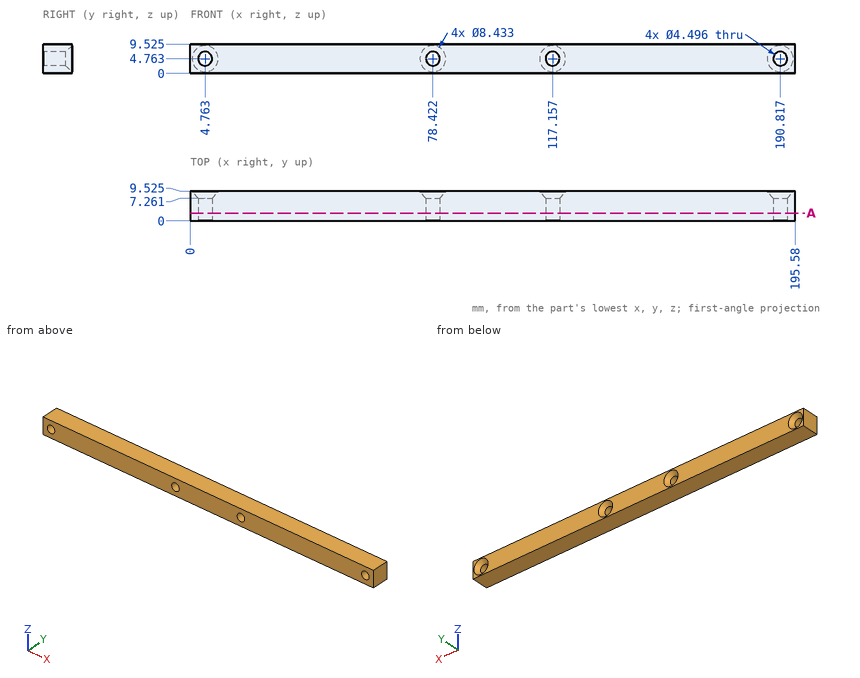
Verification items for this drawing (mm, ordinates from the low corner). Coordinates: 2 decimals unless noted, no trailing zeros. Order: outer loops, then holes, each group sorted by start corner. A loop starts at its lowest first (then second) coordinate and runs counter-clockwise, first axis right, second up. Notation, with made-up numbers: M 52.5,7.5 L 82.5,7.5 A29 ccw 82.5,40.5 Z; hole C 49.25,-25.5 d2. An arc over 180 degrees is marked long. Write each question's results on one line, items separated by ' | '.
1) Gauge pin test, flat ends, axial feed: pin 1 Ø5 at (x, z) = (22.5, 3.5) entering from -Y; pin 2 Ø5 at (x, z) = (78.42, 4.76) entering from +Y (1 decimal). Record the tip position at first contact, or that the pin passes through.
Solved:
pin 1: stops at y = 0 | pin 2: stops at y = 7.6
2) Scan lines: line 1 along X through (y, z) = (1.75, 3.5); line 2 along X through (y, z) = (5.5, 5.5) (1 decimal). Record each from-to range of solid material in increasing order. Write a range as [from, to].
Solved:
line 1: x = [0, 2.9], [6.62, 76.56], [80.28, 115.3], [119.02, 188.96], [192.68, 195.58] | line 2: x = [0, 2.6], [6.9, 76.3], [80.5, 115], [119.3, 188.7], [192.9, 195.6]
3) Section check A-A on y = 2.5. Record the cut outline in (x, z) (1 decimal).
Solved:
outline: M 0,0 L 195.6,0 L 195.6,9.5 L 0,9.5 Z; hole C 4.8,4.8 d4.5; hole C 78.4,4.8 d4.5; hole C 117.2,4.8 d4.5; hole C 190.8,4.8 d4.5
